```python
from build123d import *

# Parameters (mm, degrees)
ESQUISSE1_W             = 52
ESQUISSE1_H             = 40
BOSS_EXTRU_1_DEPTH      = 43
ESQUISSE2_W             = 48.222048012
ESQUISSE2_H             = 36
ENL_V_MAT_EXTRU_1_DEPTH = 50
ESQUISSE3_W             = 72.686110251
ESQUISSE3_H             = 50.534375484
ENL_V_MAT_EXTRU_2_DEPTH = 38
D_GAGEMENT_M61_D        = 6.6
D_GAGEMENT_M41_D        = 4.5


with BuildPart() as part:
    # Esquisse1 → Boss.-Extru.1 (new body)
    with BuildSketch(Plane.XY):
        Rectangle(ESQUISSE1_W, ESQUISSE1_H)
    extrude(amount=BOSS_EXTRU_1_DEPTH)

    # Esquisse2 → Enlèv. mat.-Extru.1 (cut)
    with BuildSketch(Plane.ZY.offset(26)):
        with Locations((26.111024006, 0)):
            Rectangle(ESQUISSE2_W, ESQUISSE2_H)
    extrude(amount=-ENL_V_MAT_EXTRU_1_DEPTH, mode=Mode.SUBTRACT)

    # Esquisse3 → Enlèv. mat.-Extru.2 (cut)
    with BuildSketch(Plane.XZ.offset(20)):
        with Locations((1.657877156, 27.267187742)):
            Rectangle(ESQUISSE3_W, ESQUISSE3_H)
    extrude(amount=-ENL_V_MAT_EXTRU_2_DEPTH, mode=Mode.SUBTRACT)

    # Dégagement M61 (through all)
    with Locations(Plane.XY.offset(2)):
        with Locations((2.997387754, 9.32052376), (-16.442863145, 9.32052376), (-16.442863145, -13.378539167), (2.997387754, -13.378539167)):
            Hole(D_GAGEMENT_M61_D / 2)

    # Dégagement M41 (through all)
    with Locations(Plane(origin=(0, 18, 0), x_dir=(-1, 0, 0), z_dir=(0, -1, 0))):
        with Locations((-4, -34.9), (-4, -23.9), (-4, -12.9), (4, -23.9)):
            Hole(D_GAGEMENT_M41_D / 2)


solid = part.part
```
Work out the finished part from the listing and answer in its coordinate system (mm). A direction names the side the tool comes from. Round coordinates to 2 decimals unless told otherwise and drop trailing zeros. Loops run counter-clockwise (first coordinate to the right, second up) from the corner with the lowest first, then second, coordinate; pieces in that order, holes last. Notation, with made-up numbers: M 43.5,10.5 L 96.5,10.5 A32 ccw 96.5,41.5 Z; hole C 15,77 d4. An arc over 180 degrees is marked long. Use CSV: the item, a comma, the result in double quotes.
Q1. Section B-B, the plane z = 12.9 is taken. Determine the outline of the cut face in (x, y), then the cut area to 3 significant figures.
Determined:
outline,"M -26,18 L 1.75,18 L 1.75,20 L -26,20 Z; M 6.25,18 L 26,18 L 26,20 L 6.25,20 Z"
area,"95.0 mm2"
Q2. Section A-A, the plane x = -4 is taken. Determine the outline of the cut face in (y, z).
Determined:
outline,"M -20,0 L 20,0 L 20,21.65 L 18,21.65 L 18,2 L -20,2 Z; M 18,26.15 L 20,26.15 L 20,43 L 18,43 Z"
Q3. Section D-D, the plane x = -14 is taken. Determine the outline of the cut face in (y, z).
Determined:
outline,"M -20,0 L -15.6,0 L -15.6,2 L -20,2 Z; M -11.16,0 L 7.1,0 L 7.1,2 L -11.16,2 Z; M 11.54,0 L 20,0 L 20,43 L 18,43 L 18,2 L 11.54,2 Z"
Q4. Each of these flat-tipped pins is pushed along its axis until it touches: pin 1 (5.5 mm diameter, centred on x = 3, y = 9.32, fed in from -Z); pin 2 (12.5 mm diameter, centred on x = 11.5, z = 25, fed in from -Y); pin 3 (10.5 mm diameter, centred on x = 3, y = -13.38, fed in from +Z). Where does it stop, or does it pass through?
Determined:
pin 1,"through"
pin 2,"y = 18"
pin 3,"z = 2"
Q5. Consider L1, parallel to X at y = 19.3, z = 23.9; L2, parallel to Z at x = 4, y = 19.15; L3, parallel to X at y = 19.4, z = 34.9. Determine where each line is inside the solid, lowest interval first.
Determined:
L1,"-26 to -6.25, -1.75 to 1.75, 6.25 to 26"
L2,"0 to 10.65, 15.15 to 21.65, 26.15 to 32.65, 37.15 to 43"
L3,"-26 to 1.75, 6.25 to 26"
Q6. A tool of negligible diameter and unlimited length cuts with its end or side. For faces 1 (the flat face through (0, -1, 2)), 2 (the cylindrical face through (5.038, 19.014, 14.896)), from which of +Z, -Z, +X, -X, +Y, -Y can it reach the whole face along a straight path? Write none if from no direction.
Determined:
face 1,"+Z, +X, -X, -Y"
face 2,"+Y, -Y"
Q7. Section C-C, the plane y = -15 is taken. Determine the outline of the cut face in (x, z).
Determined:
outline,"M -26,0 L -19.32,0 L -19.32,2 L -26,2 Z; M -13.57,0 L 0.12,0 L 0.12,2 L -13.57,2 Z; M 5.87,0 L 26,0 L 26,2 L 5.87,2 Z"
Q8. The mould has two halves that part along Z. Classify faces 3 (the cylindrical face through (-2.79, 19.014, 22.003)), 4 (the flat face through (-26, 19, 12)), 5 (the flat face through (0, 19, 43)): pulls with the +Z half, pulls with the -Z half, needs draft (parallel to the pull), parting line crosses it, or undercut.
Determined:
face 3,"undercut"
face 4,"needs draft"
face 5,"pulls with the +Z half"
